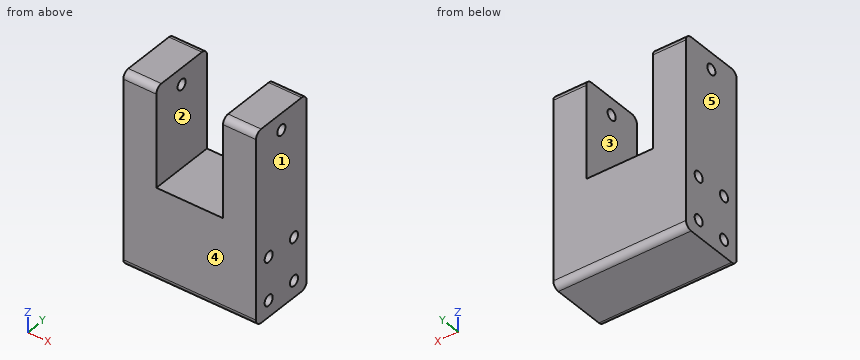
Autodesk Inventor part; units mm, degrees
ref_plane "作業平面1" through (-10.1, 0, 0) normal (-1, 0, 0) x (0, 0, 1)
ref_plane "YZ Plane" through (0, 0, 0) normal (1, 0, 0) x (0, 1, 0)
ref_plane "XZ Plane" through (0, 0, 0) normal (0, 1, 0) x (-1, 0, 0)
sketch "スケッチ1" plane through (0, 0, 0) normal (1, 0, 0) x (0, 1, 0)
  line L0 (0, 0) -> (37.4755, 0)
  line L1 (37.4755, 0) -> (37.4755, -20)
  line L2 (37.4755, -20) -> (0, -20)
  line L3 (0, -20) -> (0, 0)
  line L4 (9.6981, 10) -> (29.6981, 10)
  line L5 (29.6981, 10) -> (29.6981, -48)
  line L6 (29.6981, -48) -> (9.6981, -48)
  line L7 (9.6981, -48) -> (9.6981, 10)
  circle A0 centre (24.6981, -30) radius 1.6
  circle A1 centre (14.6981, -30) radius 1.6
  circle A2 centre (24.6981, -43) radius 1.6
  circle A3 centre (14.6981, -43) radius 1.6
  circle A4 centre (19.6981, 5) radius 1.6
  point P0 (29.6981, -20)
  point P1 (9.6981, -20)
  dimension "d0" = 20
  dimension "d1" = 10
  dimension "d2" = 3.2
  dimension "d3" = 3.2
  dimension "d4" = 3.2
  dimension "d5" = 3.2
  dimension "d6" = 10
  dimension "d7" = 10
  dimension "d8" = 13
  dimension "d9" = 0
  dimension "d10" = 0
  dimension "d11" = 13
  dimension "d12" = 5
  dimension "d13" = 10
  dimension "d14" = 5
  dimension "d15" = 5
  dimension "d16" = 3.2
  dimension "d17" = 5
  dimension "d18" = 10
extrude "押し出し1" add sketch "スケッチ1" along normal blind 10 contours L7 L4 L5 L0 | L0 L5 L2 L7 | L2 L5 L6 L7
extrude "押し出し2" add sketch "スケッチ1" against normal blind 10.1 contours L2 L5 L6 L7
ref_plane "作業平面1" through (-10.1, 0, 0) normal (-1, 0, 0) x (0, 0, 1)
mirror "ミラー1" about plane through (-10.1, 0, 0) normal (-1, 0, 0)
fillet "フィレット1" radius 2 6 edges at (5, 29.6981, 10) (5, 9.6981, 10) (-25.2, 29.6981, 10) (-25.2, 9.6981, 10) (-10.1, 29.6981, -48) (-10.1, 9.6981, -48)
equation "\"d11\" = d8"
properties part number "dribl-v1-3DP-cc-f-2" material "ABS プラスチック"
The listing builds one solid part. Answer for the finished solid, in the listing's coordinates (mm). Face numbers are marked on the shaded views. A direction names the side the tool comes from. Coordinates: 2 decimals unless noted, no trailing zeros. Loops run counter-clockwise (first coordinate to the right, second up) from the corner with the lowest first, then second, coordinate; pieces in that order, holes last. Notation, with made-up numbers: (-38.75, -29) -> (-8.75, -29) arc R6 ccw to (-8.75, -25) -> close; hole circle Ø1 at (67, 70). An arc over 180 degrees is marked (long way). Use one line per item in the form item = value. Start each with the question number.
Item 1: Consider L1, parallel to Z at x = -5, y = 14.5; L2, parallel to X at y = 18, z = -4; L3, parallel to Z at x = -2, y = 14. Determine where each line is inside the solid, lowest interval first. Write a range as [from, to].
Item 2: A tool of negligible diameter and unlimited length cuts with its end or side. For the marked faces 1 and 2, from which of +Z, -Z, +X, -X, +Y, -Y can it reach the whole face along a straight path? Write none if from no direction.
Item 3: The part is cut by section C-C on z = -43. Determine the outline of the cut face in (x, y).
Item 4: A flat-ended cylindrical pin translates along its axis: pin 1 Ø2.5 at (y, z) = (19.7, 5) entering from +X. Find the tip coordinate at first contact, or state that the pin passes through.
Item 5: The part is cut by section A-A on z = -10. Determine the outline of the cut face in (x, y).
Item 6: The part is cut by section B-B on x = -5. Determine the outline of the cut face in (y, z).
Item 7: The part is cut by section D-D on z = 5. Determine the outline of the cut face in (x, y).
Item 8: The mould has two halves that part along X. Classify the marked faces 3, 4 and 5: released by +X, released by -X, zero draft, split by the parting line, or undercut.
Answer key:
q1.L1 = [-48, -44.59], [-41.41, -31.59], [-28.41, -20]
q1.L2 = [-30.2, -20.2], [0, 10]
q1.L3 = [-48, -44.44], [-41.56, -31.44], [-28.56, -20]
q2.face_1 = +Z, -Z, +X, +Y, -Y
q2.face_2 = +Z, +Y, -Y
q3.outline = (-30.2, 9.7) -> (10, 9.7) -> (10, 13.1) -> (-30.2, 13.1) -> close; (-30.2, 16.3) -> (10, 16.3) -> (10, 23.1) -> (-30.2, 23.1) -> close; (-30.2, 26.3) -> (10, 26.3) -> (10, 29.7) -> (-30.2, 29.7) -> close
q4.pin_1 = through
q5.outline = (-30.2, 9.7) -> (-20.2, 9.7) -> (-20.2, 29.7) -> (-30.2, 29.7) -> close; (0, 9.7) -> (10, 9.7) -> (10, 29.7) -> (0, 29.7) -> close
q6.outline = (9.7, -46) arc R2 ccw to (11.7, -48) -> (27.7, -48) arc R2 ccw to (29.7, -46) -> (29.7, -20) -> (9.7, -20) -> close; hole circle Ø3.2 at (14.7, -43); hole circle Ø3.2 at (14.7, -30); hole circle Ø3.2 at (24.7, -43); hole circle Ø3.2 at (24.7, -30)
q7.outline = (-30.2, 9.7) -> (-20.2, 9.7) -> (-20.2, 18.1) -> (-30.2, 18.1) -> close; (-30.2, 21.3) -> (-20.2, 21.3) -> (-20.2, 29.7) -> (-30.2, 29.7) -> close; (0, 9.7) -> (10, 9.7) -> (10, 18.1) -> (0, 18.1) -> close; (0, 21.3) -> (10, 21.3) -> (10, 29.7) -> (0, 29.7) -> close
q8.face_3 = undercut
q8.face_4 = zero draft
q8.face_5 = released by -X
